Build history of the part. All positions in model axes, mm. A direction names the side the tool comes from. Coordinates: 2 decimals unless noted, no trailing zeros. Order: outer loops, then holes, each group sorted by start corner. A loop starts at its lowest first (then second) coordinate and runs counter-clockwise, first axis right, second up. Notation, with made-up numbers: (55.5, -16.5) - (97.5, -16.5) arc R19 ccw to (97.5, 0.5) - close; hole circle Ø6 at (18, -32.75). An arc over 180 degrees is marked (long way). Return JSON: item names as keys, results as strings.
from build123d import *

# Parameters (mm, degrees)
SKETCH2_W           = 1500
SKETCH2_H           = 1500
BOSS_EXTRUDE1_DEPTH = 10
BOSS_EXTRUDE2_DEPTH = 110
BOSS_EXTRUDE3_DEPTH = 10


with BuildPart() as part:
    # Sketch2 → Boss-Extrude1 (new body)
    with BuildSketch(Plane(origin=(0, 0, 0), x_dir=(1, 0, 0), z_dir=(0, 1, 0))):
        Rectangle(SKETCH2_W, SKETCH2_H)
    extrude(amount=BOSS_EXTRUDE1_DEPTH)

    # Sketch3 → Boss-Extrude2 (add)
    with BuildSketch(Plane(origin=(0, 10, 0), x_dir=(1, 0, 0), z_dir=(0, 1, 0))):
        with BuildLine():
            ThreePointArc((750, -600), (-204.594154602, -204.594154602), (-600, 750))
            Line((-600, 750), (-620, 750))
            ThreePointArc((-620, 750), (-218.736290226, -218.736290226), (750, -620))
            Line((750, -620), (750, -600))
        make_face()
        with BuildLine():
            Line((620, 750), (600, 750))
            ThreePointArc((600, 750), (643.933982822, 643.933982822), (750, 600))
            Line((750, 600), (750, 620))
            ThreePointArc((750, 620), (658.076118446, 658.076118446), (620, 750))
        make_face()
    extrude(amount=BOSS_EXTRUDE2_DEPTH)

    # Sketch4 → Boss-Extrude3 (add)
    with BuildSketch(Plane(origin=(0, 10, 0), x_dir=(1, 0, 0), z_dir=(0, 1, 0))):
        Polygon((-391.421356236, 636.86291501), (-419.705627484, 608.578643763), (-391.421356236, 580.294372515), (-363.137084989, 608.578643763), align=None)
        Polygon((-191.421356236, 636.86291501), (-219.705627484, 608.578643763), (-191.421356236, 580.294372515), (-163.137084989, 608.578643763), align=None)
        Polygon((8.578643763, 636.86291501), (-19.705627484, 608.578643763), (8.578643763, 580.294372515), (36.862915011, 608.578643763), align=None)
        Polygon((208.578643763, 636.86291501), (180.294372516, 608.578643763), (208.578643763, 580.294372515), (236.862915011, 608.578643763), align=None)
        Polygon((408.578643763, 636.86291501), (380.294372515, 608.578643763), (408.578643763, 580.294372515), (436.86291501, 608.578643763), align=None)
        Polygon((-191.421356236, 436.86291501), (-219.705627484, 408.578643763), (-191.421356236, 380.294372515), (-163.137084989, 408.578643763), align=None)
        Polygon((8.578643763, 436.86291501), (-19.705627484, 408.578643763), (8.578643763, 380.294372515), (36.862915011, 408.578643763), align=None)
        Polygon((208.578643763, 436.86291501), (180.294372516, 408.578643763), (208.578643763, 380.294372515), (236.862915011, 408.578643763), align=None)
        Polygon((408.578643763, 436.86291501), (380.294372515, 408.578643763), (408.578643763, 380.294372515), (436.86291501, 408.578643763), align=None)
        Polygon((-191.421356236, 236.86291501), (-219.705627484, 208.578643763), (-191.421356236, 180.294372515), (-163.137084989, 208.578643763), align=None)
        Polygon((8.578643763, 236.86291501), (-19.705627484, 208.578643763), (8.578643763, 180.294372515), (36.862915011, 208.578643763), align=None)
        Polygon((208.578643763, 236.86291501), (180.294372516, 208.578643763), (208.578643763, 180.294372515), (236.862915011, 208.578643763), align=None)
        Polygon((408.578643763, 236.86291501), (380.294372515, 208.578643763), (408.578643763, 180.294372515), (436.86291501, 208.578643763), align=None)
        Polygon((-191.421356236, 36.86291501), (-219.705627484, 8.578643763), (-191.421356236, -19.705627485), (-163.137084989, 8.578643763), align=None)
        Polygon((8.578643763, 36.86291501), (-19.705627484, 8.578643763), (8.578643763, -19.705627485), (36.862915011, 8.578643763), align=None)
        Polygon((208.578643763, 36.86291501), (180.294372516, 8.578643763), (208.578643763, -19.705627485), (236.862915011, 8.578643763), align=None)
        Polygon((408.578643763, 36.86291501), (380.294372515, 8.578643763), (408.578643763, -19.705627485), (436.86291501, 8.578643763), align=None)
        Polygon((8.578643763, -163.13708499), (-19.705627484, -191.421356237), (8.578643763, -219.705627485), (36.862915011, -191.421356237), align=None)
        Polygon((208.578643763, -163.13708499), (180.294372516, -191.421356237), (208.578643763, -219.705627485), (236.862915011, -191.421356237), align=None)
        Polygon((408.578643763, -163.13708499), (380.294372515, -191.421356237), (408.578643763, -219.705627485), (436.86291501, -191.421356237), align=None)
        Polygon((-391.421356236, 436.86291501), (-419.705627484, 408.578643763), (-391.421356236, 380.294372515), (-363.137084989, 408.578643763), align=None)
        Polygon((-391.421356236, 236.86291501), (-419.705627484, 208.578643763), (-391.421356236, 180.294372515), (-363.137084989, 208.578643763), align=None)
        Polygon((208.578643763, -363.13708499), (180.294372516, -391.421356237), (208.578643763, -419.705627485), (236.862915011, -391.421356237), align=None)
        Polygon((408.578643763, -363.13708499), (380.294372515, -391.421356237), (408.578643763, -419.705627485), (436.86291501, -391.421356237), align=None)
        Polygon((608.578643763, 636.86291501), (580.294372515, 608.578643763), (608.578643763, 580.294372515), (636.86291501, 608.578643763), align=None)
        Polygon((608.578643763, 436.86291501), (580.294372515, 408.578643763), (608.578643763, 380.294372515), (636.86291501, 408.578643763), align=None)
        Polygon((608.578643763, 236.86291501), (580.294372515, 208.578643763), (608.578643763, 180.294372515), (636.86291501, 208.578643763), align=None)
        Polygon((608.578643763, 36.86291501), (580.294372515, 8.578643763), (608.578643763, -19.705627485), (636.86291501, 8.578643763), align=None)
        Polygon((608.578643763, -163.13708499), (580.294372515, -191.421356237), (608.578643763, -219.705627485), (636.86291501, -191.421356237), align=None)
        Polygon((608.578643763, -363.13708499), (580.294372515, -391.421356237), (608.578643763, -419.705627485), (636.86291501, -391.421356237), align=None)
    extrude(amount=BOSS_EXTRUDE3_DEPTH)


solid = part.part
1. Drop flat-ended pins along their axis: pin 1 (17 mm diameter, centred on x = 197, z = -613.5, fed in from +Y); pin 2 (1 mm diameter, centred on x = 588, y = 42.5, fed in from +Z); pin 3 (1.5 mm diameter, centred on y = 65.5, z = -184.5, fed in from +X). Give the stop position or say it passes through.
Check values:
{"pin 1": "y = 20", "pin 2": "z = 610.45", "pin 3": "x = -475.5"}
2. Cut at B-B on z = 50. Give the cut face in (x, y).
Check values:
{"outline": "(-750, 0) - (750, 0) - (750, 10) - (-337.43, 10) - (-337.43, 120) - (-362.16, 120) - (-362.16, 10) - (-750, 10) - close"}
3. Mould opens along Z. For faces 1 (the flat face through (608, 20, 391)), 2 (the flat face through (8, 20, -9)), 3 (the flat face through (608, 20, -209)), 4 (the flat face through (-4, 2, -750)) say: pulls with the +Z half, pulls with the -Z half, needs draft (parallel to the pull), parting line crosses it, or undercut.
Check values:
{"face 1": "undercut", "face 2": "needs draft", "face 3": "undercut", "face 4": "pulls with the -Z half"}
4. Cut at C-C on x = -524. Give the cut face in (y, z), plus the area to 3 significant figures.
Check values:
{"outline": "(0, -750) - (10, -750) - (10, -303.43) - (120, -303.43) - (120, -246.19) - (10, -246.19) - (10, 750) - (0, 750) - close", "area": "21,300 mm²"}
5. Tool access for faces 5 (the flat face through (216, 10, -234)), 6 (the cylindrical face through (-229.329, 64.23, 208.026)), 7 (the flat face through (-192, 20, -609)), 8 (the flat face through (-192, 20, -209)): list every direction of +Z, -Z, +X, -X, +Y, -Y with a clear straight run to the whole face (end or side of a thin tool).
Check values:
{"face 5": "+Y", "face 6": "+Z, -X, +Y", "face 7": "-Z, +Y", "face 8": "-Z, +X, +Y"}
6. Cut at A-A on y = 85.5. Give the cut face in (x, z).
Check values:
{"outline": "(-620, -750) - (-600, -750) arc R1350 cw to (750, 600) - (750, 620) arc R1370 ccw to start; (600, -750) - (620, -750) arc R130 cw to (750, -620) - (750, -600) arc R150 ccw to start"}
7. Probe L1, parallel to Y at x = 165.5, z = 86.5; L2, parallel to Y at x = 611.5, z = -29; L3, parallel to X at y = 62, z = -644. List the from-to ranges inside material, lowest first.
Check values:
{"L1": "0 to 10", "L2": "0 to 20", "L3": "-615.89 to -595.83, 643.87 to 674.74"}
